from build123d import *

# Parameters (mm, degrees)
F1_W      = 47.35
F1_H      = 47.35
F2_DEPTH  = 2
F3_DEPTH  = 107.95
F4_R      = 6.35
F7_DEPTH  = 107.951
F8_R      = 6.35
F9_DEPTH  = 25
F10_R     = 2
F11_W     = 2
F11_H     = 12.7
F12_DEPTH = 107.951
F13_DEPTH = 25


# Not quite as in the source:
# - a feature names something its author has since deleted; it is built from what else it names


with BuildPart() as f2:
    # F1 (on Right) → F2 (new body)
    with BuildSketch(Plane.YZ):
        Rectangle(F1_W, F1_H)
        Polygon((19.3428993274, 21.675), (21.675, 21.675), (21.675, 19.3428993274), (21.675, -19.3428993274), (21.675, -21.675), (19.3428993274, -21.675), (-19.3428993274, -21.675), (-21.675, -21.675), (-21.675, -19.3428993274), (-21.675, 19.3428993274), (-21.675, 21.675), (-19.3428993274, 21.675), align=None, mode=Mode.SUBTRACT)
        Polygon((21.675, 19.3428993274), (19.3428993274, 21.675), (-19.3428993274, 21.675), (-21.675, 19.3428993274), (-21.675, -19.3428993274), (-19.3428993274, -21.675), (19.3428993274, -21.675), (21.675, -19.3428993274), align=None)
        Polygon((-19.3428993274, -21.675), (-21.675, -19.3428993274), (-21.675, -21.675), align=None)
        Polygon((21.675, -21.675), (21.675, -19.3428993274), (19.3428993274, -21.675), align=None)
        Polygon((21.675, 19.3428993274), (21.675, 21.675), (19.3428993274, 21.675), align=None)
        Polygon((-21.675, 19.3428993274), (-19.3428993274, 21.675), (-21.675, 21.675), align=None)
    extrude(amount=F2_DEPTH)

    # F1 (on Right) → F3 (join)
    with BuildSketch(Plane.YZ):
        Rectangle(F1_W, F1_H)
        Polygon((19.3428993274, 21.675), (21.675, 21.675), (21.675, 19.3428993274), (21.675, -19.3428993274), (21.675, -21.675), (19.3428993274, -21.675), (-19.3428993274, -21.675), (-21.675, -21.675), (-21.675, -19.3428993274), (-21.675, 19.3428993274), (-21.675, 21.675), (-19.3428993274, 21.675), align=None, mode=Mode.SUBTRACT)
        Polygon((21.675, 19.3428993274), (21.675, 21.675), (19.3428993274, 21.675), align=None)
        Polygon((21.675, -21.675), (21.675, -19.3428993274), (19.3428993274, -21.675), align=None)
        Polygon((-19.3428993274, -21.675), (-21.675, -19.3428993274), (-21.675, -21.675), align=None)
        Polygon((-21.675, 19.3428993274), (-19.3428993274, 21.675), (-21.675, 21.675), align=None)
    extrude(amount=F3_DEPTH)

    # F4 (on face) → F7 (cut, through all)
    with BuildSketch(Plane.YZ):
        Circle(F4_R)
    extrude(amount=F7_DEPTH, mode=Mode.SUBTRACT)

    # F8 (on face) → F9 (cut)
    with BuildSketch(Plane(origin=(0, 23.675, 0), x_dir=(-1, 0, 0), z_dir=(0, 1, 0))):
        with Locations((-94.95, 0)):
            Circle(F8_R)
    extrude(amount=-F9_DEPTH, mode=Mode.SUBTRACT)

    # F10
    f10_edges = [f2.edges().sort_by_distance(p)[0] for p in [
        (53.975, -23.675, 23.675),
        (53.975, 23.675, 23.675),
        (53.975, 23.675, -23.675),
        (53.975, -23.675, -23.675),
    ]]
    fillet(f10_edges, radius=F10_R)

    # F11 (on face) → F12 (cut, through all)
    with BuildSketch(Plane.YZ.offset(107.95)):
        with Locations((22.675, 0)):
            Rectangle(F11_W, F11_H)
    extrude(amount=-F12_DEPTH, mode=Mode.SUBTRACT)

    # F1 (on Right) → F13 (cut)
    with BuildSketch(Plane.YZ):
        Polygon((21.675, 19.3428993274), (19.3428993274, 21.675), (-19.3428993274, 21.675), (-21.675, 19.3428993274), (-21.675, -19.3428993274), (-19.3428993274, -21.675), (19.3428993274, -21.675), (21.675, -19.3428993274), align=None)
    extrude(amount=F13_DEPTH, mode=Mode.SUBTRACT)


solid = f2.part
Can you work these out from the model? Positions are in its coordinate system, mm. A direction names the side the tool comes from. Coordinates: 2 decimals unless noted, no trailing zeros. Write each loop counter-clockwise with the first axis right and the second up, starting at its lowest first coordinate (ties: lowest second). Pieces come first, ordered by that corner, then holes. Notation, with made-up numbers: (67.25, 85) -> (76.25, 85) arc R20 cw to (76.25, 113) -> close; hole circle Ø8 at (63.5, -6). An arc over 180 degrees is marked (long way). Write each question's results on one line, items separated by ' | '. Start each with the question number.
Q1. Imagine slicing it at C-C (x = 45). Write out the boundary of the cut face in (y, z) (3 decimals).
Q2. Imagine slicing it at A-A (y = 18). Write out the boundary of the cut face in (x, z) (3 decimals), then the cut area to 3 significant figures.
Q3. Imagine slicing it at D-D (z = -4). Write out the boundary of the cut face in (x, y) (3 decimals).
Q4. We'd pull the mould along Z, two halves only. Please class faces 1 (the face through (53, 0, -21.675)), 2 (the face through (53.219, 23.074, 23.105)), 3 (the face through (54.731, -23.105, -23.074)): +Z half, -Z half, draft (parallel to the pull), parting line (faces both ways), or undercut.
Q5. On a 3-axis mill with a long thin cutter (end or side, diameter ignored), from which of +Z, -Z, +X, -X, +Y, -Y can I reach the whole of each face in a straight line? I mean faces 4 (the face through (55, 23, -6.35)), 5 (the face through (0, -23, 0)), 6 (the face through (53.22, -20.53, 20.49)). Say none if no direction works.
Q6. If I drill on probe 1 along Y at (x, z) = (68.5, 12) (3 decimals); probe 2 along Y at (x, z) = (94.5, 0.5) (3 decimals), over which ranges is the centre line in solid material (lowest first)?
Q7. I'm going to push flat-ended pins straight in: pin 1 (1 mm diameter, centred on x = 78, y = 23, fed in from -Z); pin 2 (10 mm diameter, centred on y = -13.5, z = -1.5, fed in from -X); pin 3 (0.6 mm diameter, centred on x = 69, y = 23, fed in from +Z). Where does each tip first touch, or does it pass through?
Taken from the geometry:
1) outline: (-23.675, -21.675) arc R2 ccw to (-21.675, -23.675) -> (21.675, -23.675) arc R2 ccw to (23.675, -21.675) -> (23.675, -6.35) -> (21.675, -6.35) -> (21.675, -19.343) -> (19.343, -21.675) -> (-19.343, -21.675) -> (-21.675, -19.343) -> (-21.675, 19.343) -> (-19.343, 21.675) -> (19.343, 21.675) -> (21.675, 19.343) -> (21.675, 6.35) -> (23.675, 6.35) -> (23.675, 21.675) arc R2 ccw to (21.675, 23.675) -> (-21.675, 23.675) arc R2 ccw to (-23.675, 21.675) -> close
2) outline: (0, -23.675) -> (107.95, -23.675) -> (107.95, -21.675) -> (0, -21.675) -> close; (0, 21.675) -> (107.95, 21.675) -> (107.95, 23.675) -> (0, 23.675) -> close | area: 432 mm^2
3) outline: (0, -23.675) -> (107.95, -23.675) -> (107.95, -21.675) -> (0, -21.675) -> close
4) face 1: undercut | face 2: +Z half | face 3: -Z half
5) face 4: +X, -X, +Y | face 5: +Z, -Z, -X, +Y, -Y | face 6: +X, -X
6) probe 1: y = -23.675 to -21.675, 21.675 to 23.675 | probe 2: y = -23.675 to -21.675
7) pin 1: stops at z = -23.5 | pin 2: passes through | pin 3: stops at z = 23.39
